Read the model definition and answer for the solid it produces. Units are mm, in the model's axes. A direction names the side the tool comes from. Coordinates: 2 decimals unless noted, no trailing zeros. Order: outer loops, then holes, each group sorted by start corner. A loop starts at its lowest first (then second) coordinate and runs counter-clockwise, first axis right, second up. Notation, with made-up numbers: (43.5, 5.25) -> (50.5, 5.25) arc R18 cw to (50.5, 40.25) -> close; hole circle Ø4 at (0.25, 38.5). An arc over 180 degrees is marked (long way). Answer as a JSON object with one key per item and string values. Group by question number.
1) Given pin 1 (4.5 mm diameter, centred on y = -5.5, z = -3.5, fed in from -X); pin 2 (1 mm diameter, centred on x = 84, y = -18, fed in from -Z); pin 3 (4 mm diameter, centred on x = 47.5, z = 37.5, fed in from -Y); pin 4 (4 mm diameter, centred on x = 35.5, y = -21, fed in from +Z), each flat-ended and moving along its own axis, determine where each tip first touches the part or whether it passes through.
2) Section D-D on y = -36 is taken. Determine the outline of the cut face in (x, z).
3) Section B-B on y = -24.5 is taken. Determine the outline of the cut face in (x, z), and give its area (3 significant figures).
4) A tool of negligible diameter and unlimited length cuts with its end or side. For faces 4 (the flat face through (74, -1, -32)), 5 (the flat face through (74, -3, -35)), 6 (the flat face through (72, -1, 42)), from which of +Z, -Z, +X, -X, +Y, -Y can it reach the whole face along a straight path? Write none if from no direction.
5) Consider L1, parallel to Z at x = 73, y = -1.85; L2, parallel to X at y = -24.5, z = -28; L3, parallel to Z at x = 133, y = -1.85. Determine where each line is inside the solid, lowest interval first.
6) Determine the mould class of faces 1 (the cylindrical face through (113, -15, 0)), 2 (the flat face through (146, -16, -1)), 3 (the flat face through (74, -1, -42)) for opening direction X: released by +X, released by -X, zero draft, split by the parting line, or undercut.
7) Section C-C on z = 0 is taken. Determine the outline of the cut face in (x, y), and give its area (3 significant figures).
Autodesk Inventor part; units mm, degrees
ref_plane "YZ Plane" through (0, 0, 0) normal (1, 0, 0) x (0, 1, 0)
ref_plane "XZ Plane" through (0, 0, 0) normal (0, 1, 0) x (-1, 0, 0)
ref_plane "XY Plane" through (0, 0, 0) normal (0, 0, 1) x (1, 0, 0)
sketch "Szkic1" plane through (0, 0, 0) normal (1, 0, 0) x (0, 1, 0)
  circle A0 centre (0, 0) radius 42
  dimension "d0" = 84
extrude "Wyciągnięcie proste1" add sketch "Szkic1" along normal blind 146
ref_plane "Płaszczyzna konstrukcyjna1" through (3, 0, 0) normal (-1, 0, 0) x (0, 0, 1)
sketch "Szkic2" plane through (3, 0, 0) normal (-1, 0, 0) x (0, 0, 1)
  point P0 (0, 0)
sketch "Szkic3" plane through (3, 0, 0) normal (-1, 0, 0) x (0, 0, 1)
  circle A0 centre (0, 0) radius 17
  circle A1 centre (0, 0) radius 15
  arc A2 (-17.4356, 36) -> (17.4356, 36) centre (0, 0) ccw
  line L0 (17.4356, 36) -> (-17.4356, 36)
  dimension "d4" = 34
  dimension "d5" = 30
  dimension "d10" = 80
sketch "Szkic4" plane through (0, 0, 0) normal (-1, 0, 0) x (0, 0, 1)
  circle A0 centre (0, 0) radius 42
  circle A1 centre (0, 0) radius 4.5
  circle A2 centre (10, 0) radius 2
  circle A3 centre (-10, 0) radius 2
  dimension "d6" = 9
extrude "Wyciągnięcie proste2" cut sketch "Szkic4" against normal blind 146 contours A1 | A2 | A3
extrude "Wyciągnięcie proste3" cut sketch "Szkic3" against normal blind 140
ref_plane "Płaszczyzna konstrukcyjna2" through (63, 0, 0) normal (-1, 0, 0) x (0, 0, 1)
sketch "Szkic6" plane through (63, 0, 0) normal (-1, 0, 0) x (0, 0, 1)
  circle A0 centre (0, 0) radius 17
extrude "Wyciągnięcie proste4" cut sketch "Szkic6" against normal blind 20
sketch "Szkic7" plane through (0, 0, 0) normal (-1, 0, 0) x (0, 0, 1)
  circle A0 centre (-10, 0) radius 2
  circle A1 centre (10, 0) radius 2
  circle A2 centre (0, 0) radius 4.5
  circle A3 centre (0, 0) radius 42
  point P0 (42, 0)
ref_plane "Płaszczyzna konstrukcyjna3" through (0, 0, 42) normal (0, 0, 1) x (1, 0, 0)
sketch "Szkic8" plane through (0, 0, 42) normal (0, 0, 1) x (1, 0, 0)
  line L0 (0, -4.5) -> (0, 4.5)
  line L1 (146, 3) -> (0, 3)
  line L2 (0, 3) -> (0, -3)
  line L3 (0, -3) -> (146, -3)
  line L4 (146, -3) -> (146, 3)
  line L5 (146, 3) -> (0, -3) construction
  line L6 (0, 3) -> (146, -3) construction
  point P0 (0, 0)
  point P1 (73, 0)
  dimension "d16" = 6
extrude "Wyciągnięcie proste5" add sketch "Szkic8" against normal blind 10
sketch "Szkic9" plane through (0, 0, 0) normal (-1, 0, 0) x (0, 0, 1)
  line L0 (42, 3) -> (42, -3)
  line L1 (42, 3) -> (41.8927, 3)
  arc A0 (41.8927, 3) -> (41.8927, -3) centre (0, 0) ccw
  line L2 (42, -3) -> (41.8927, -3)
  circle A1 centre (0, 0) radius 4.5
  circle A2 centre (10, 0) radius 2
  circle A3 centre (-10, 0) radius 2
  point P0 (-42, 0)
ref_plane "Płaszczyzna konstrukcyjna4" through (0, 0, -42) normal (0, 0, -1) x (-1, 0, 0)
sketch "Szkic10" plane through (0, 0, -42) normal (0, 0, -1) x (-1, 0, 0)
  line L0 (-146, -3) -> (0, -3)
  line L1 (0, -3) -> (0, 3)
  line L2 (0, 3) -> (-146, 3)
  line L3 (-146, 3) -> (-146, -3)
  line L4 (-146, -3) -> (0, 3) construction
  line L5 (0, -3) -> (-146, 3) construction
  point P0 (0, 0)
  point P1 (-73, 0)
extrude "Wyciągnięcie proste6" add sketch "Szkic10" against normal blind 10
sketch "Szkic11" plane through (0, 0, 0) normal (-1, 0, 0) x (0, 0, 1)
  circle A0 centre (-10, 0) radius 2
  circle A1 centre (10, 0) radius 2
  circle A2 centre (0, 0) radius 4.5
  line L0 (-42, -3) -> (-42, 3)
  line L1 (-42, -3) -> (-41.8927, -3)
  arc A3 (-41.8927, -3) -> (41.8927, -3) centre (0, 0) ccw
  line L2 (42, -3) -> (41.8927, -3)
  line L3 (42, 3) -> (42, -3)
  line L4 (42, 3) -> (41.8927, 3)
  arc A4 (41.8927, 3) -> (-41.8927, 3) centre (0, 0) ccw
  line L5 (-42, 3) -> (-41.8927, 3)
  arc A5 (41.8927, 3) -> (-41.8927, 3) centre (0, 0) ccw
  point P0 (0, 42)
ref_plane "Płaszczyzna konstrukcyjna5" through (0, 42, 0) normal (0, 1, 0) x (-1, 0, 0)
sketch "Szkic12" plane through (0, 42, 0) normal (0, 1, 0) x (-1, 0, 0)
  circle A0 centre (-73, -36) radius 1
  circle A1 centre (-133, -36) radius 1
  circle A2 centre (-13, -36) radius 1
  circle A3 centre (-13, 36) radius 1
  circle A4 centre (-73, 36) radius 1
  circle A5 centre (-133, 36) radius 1
  point P0 (0, 0)
extrude "Wyciągnięcie proste7" cut sketch "Szkic12" against normal blind 45
ref_plane "Płaszczyzna konstrukcyjna7" through (0, 38, 0) normal (0, 1, 0) x (-1, 0, 0)
sketch "Szkic16" plane through (0, 42, 0) normal (0, 1, 0) x (-1, 0, 0)
  line L0 (-110, -6) -> (-36, -6)
  line L1 (-36, -6) -> (-36, 1)
  line L2 (-42, 6) -> (-104, 6)
  line L3 (-110, 1) -> (-110, -6)
  line L4 (-110, -6) -> (-36, 6) construction
  line L5 (-36, -6) -> (-110, 6) construction
  line L6 (-2, -15) -> (-144, -15)
  line L7 (-144, -15) -> (-144, 15)
  line L8 (-144, 15) -> (-2, 15)
  line L9 (-2, 15) -> (-2, -15)
  line L10 (-2, -15) -> (-144, 15) construction
  line L11 (-144, -15) -> (-2, 15) construction
  line L12 (-110, 1) -> (-104, 1)
  line L13 (-104, 1) -> (-104, 6)
  line L14 (-36, 1) -> (-42, 1)
  line L15 (-42, 1) -> (-42, 6)
  point P0 (0, 0)
  point P1 (-73, 0)
  dimension "d36" = 74
  dimension "d37" = 12
extrude "Wyciągnięcie proste11" cut sketch "Szkic16" against normal blind 4.25 contours L3 L12 L13 L2 L15 L14 L1 L0
sketch "Szkic17" plane through (0, 38, 0) normal (0, 1, 0) x (-1, 0, 0)
  line L0 (-110.5, -6.5) -> (-35.5, -6.5)
  line L1 (-35.5, -6.5) -> (-35.5, 6.5)
  line L2 (-35.5, 6.5) -> (-110.5, 6.5)
  line L3 (-110.5, 6.5) -> (-110.5, -6.5)
  line L4 (-110.5, -6.5) -> (-35.5, 6.5) construction
  line L5 (-35.5, -6.5) -> (-110.5, 6.5) construction
  point P0 (0, 0)
  point P1 (-73, 0)
  dimension "d40" = 75
  dimension "d41" = 13
extrude "Wyciągnięcie proste12" cut sketch "Szkic17" along normal blind 0.5
sketch "Szkic18" plane through (0, 0, 0) normal (-1, 0, 0) x (0, 0, 1)
  line L0 (42, 3) -> (42, -3)
  line L1 (42, 0) -> (-42, 0)
  line L2 (-42, 0) -> (-42, 42)
  line L3 (-42, 42) -> (42, 42)
  line L4 (42, 42) -> (42, 0)
extrude "Wyciągnięcie proste13" cut sketch "Szkic18" against normal blind 146
properties part number "v1.0L"
Worked answers:
{
 "1": {"pin 1": "stops at x = 0", "pin 2": "stops at z = -38.18", "pin 3": "stops at y = -22.44", "pin 4": "stops at z = 37.46"},
 "2": {"outline": "(0, -21.63) -> (146, -21.63) -> (146, 21.63) -> (0, 21.63) -> close; hole (3, -17.44) -> (143, -17.44) -> (143, 17.44) -> (3, 17.44) -> close"},
 "3": {"outline": "(0, -34.11) -> (146, -34.11) -> (146, 34.11) -> (0, 34.11) -> close; hole (3, -31.62) -> (143, -31.62) -> (143, 31.62) -> (3, 31.62) -> close", "area": "1,110 mm²"},
 "4": {"face 4": "+Y", "face 5": "none", "face 6": "+Z, +X, -X, +Y, -Y"},
 "5": {"L1": "z = -42 to -37, -35 to -32, 32 to 35, 37 to 42", "L2": "x = 0 to 3, 143 to 146", "L3": "z = -42 to -37, -35 to -32, -16.9 to -14.89, 14.89 to 16.9, 32 to 35, 37 to 42"},
 "6": {"face 1": "undercut", "face 2": "released by +X", "face 3": "zero draft"},
 "7": {"outline": "(0, -42) -> (146, -42) -> (146, -4.5) -> (143, -4.5) -> (143, -15) -> (83, -15) -> (83, -17) -> (143, -17) -> (143, -40) -> (3, -40) -> (3, -17) -> (63, -17) -> (63, -15) -> (3, -15) -> (3, -4.5) -> (0, -4.5) -> close", "area": "745 mm²"}
}
